```python
from build123d import *

# Parameters (mm, degrees)
F3_DEPTH  = 18.75
F4_W      = 19.4052183703
F4_H      = 18.75
F4_W_2    = 8
F5_DEPTH  = 3
F6_R      = 2.25
F7_DEPTH  = 12
F9_DEPTH  = 3.3
F11_DEPTH = 35


with BuildPart() as f3:
    # F2 (on Top) → F3 (new body)
    with BuildSketch(Plane.XY):
        Polygon((-6.6899931507, 11.2585633857), (-6.6899931507, 24.0085633857), (-5.1899931507, 24.0085633857), (-6.6899931507, 25.5085633857), (-9.6899931507, 25.5085633857), (-9.6899931507, 24.0085633857), (-9.6899931507, 11.2585633857), (-9.6899931507, -18.7414366143), (9.0600068493, -13.7414366143), (9.0600068493, 11.2585633857), (9.0600068493, 24.0085633857), (9.0600068493, 25.5085633857), (6.0600068493, 25.5085633857), (4.5600068493, 24.0085633857), (6.0600068493, 24.0085633857), (6.0600068493, 11.2585633857), align=None)
    extrude(amount=F3_DEPTH)

    # F4 (on face) → F5 (join)
    with BuildSketch(Plane(origin=(4.0225987819, -15.0847454323, 0), x_dir=(0.9662349396, 0.2576626506, 0), z_dir=(0.2576626506, -0.9662349396, 0))):
        with Locations((-4.4891689949, 9.375)):
            Rectangle(F4_W, F4_H)
        with Locations((-18.1917781801, 9.375)):
            Rectangle(F4_W_2, F4_H)
        with Locations((9.2134401902, 9.375)):
            Rectangle(F4_W_2, F4_H)
    extrude(amount=F5_DEPTH)

    # F6 (on face) → F7 (cut)
    with BuildSketch(Plane(origin=(4.7955867336, -17.9834502511, 0), x_dir=(0.9662349396, 0.2576626506, 0), z_dir=(0.2576626506, -0.9662349396, 0))):
        with Locations((7.2134401902, 9.375)):
            Circle(F6_R)
        with Locations((-16.1917781801, 9.375)):
            Circle(F6_R)
    extrude(amount=-F7_DEPTH, mode=Mode.SUBTRACT)

    # F8 (on face) → F9 (cut)
    with BuildSketch(Plane(origin=(4.0225987819, -15.0847454323, 0), x_dir=(0.9662349396, 0.2576626506, 0), z_dir=(0.2576626506, -0.9662349396, 0))):
        Polygon((5.2134401902, 5.775), (9.2919011593, 5.775), (11.3703621284, 9.375), (9.2919011593, 12.975), (5.2134401902, 12.975), align=None)
        Polygon((5.1349792211, 5.775), (5.2134401902, 5.775), (5.2134401902, 12.975), (5.1349792211, 12.975), (3.0565182521, 9.375), align=None)
        Polygon((-18.2702391492, 5.775), (-14.1917781801, 5.775), (-14.1917781801, 12.975), (-18.2702391492, 12.975), (-20.3487001183, 9.375), align=None)
        Polygon((-14.1917781801, 12.975), (-14.1917781801, 5.775), (-14.113317211, 5.775), (-12.0348562419, 9.375), (-14.113317211, 12.975), align=None)
    extrude(amount=-F9_DEPTH, mode=Mode.SUBTRACT)

    # F10 (on face) → F11 (join)
    with BuildSketch(Plane(origin=(0, 0, 0), x_dir=(1, 0, 0), z_dir=(0, 0, -1))):
        Polygon((9.0600068493, -8.2585633857), (-9.6899931507, -8.2585633857), (-9.6899931507, -25.5085633857), (-6.6899931507, -25.5085633857), (-5.1899931507, -24.0085633857), (-6.6899931507, -24.0085633857), (-6.6899931507, -11.2585633857), (6.0600068493, -11.2585633857), (6.0600068493, -24.0085633857), (4.5600068493, -24.0085633857), (6.0600068493, -25.5085633857), (9.0600068493, -25.5085633857), align=None)
    extrude(amount=F11_DEPTH)


solid = f3.part
```
Part model, mm, in its own coordinate system. A direction names the side the tool comes from. Round coordinates to 2 decimals unless told otherwise and drop trailing zeros. Loops run counter-clockwise (first coordinate to the right, second up) from the corner with the lowest first, then second, coordinate; pieces in that order, holes last.
Item 1: Mould opens along Y. For faces 1 (the face through (8.046, -4.697, 9.406)), 2 (the face through (0, 11, -35)), 3 (the face through (-5.95, 24.77, -7.75)), 4 (the face through (7.547, -12.461, 7.6)) say: +Y half, -Y half, draft (parallel to the pull), parting line (faces both ways), or undercut.
Item 2: Cut at A-A, the plane z = 15. Give the cut face in (x, y), then the cut area to 3 significant figures.
Item 3: Drop flat-ended pins along their axis: P1, Ø12, axis at y = -12, z = -9, coming from the -X side; P2, Ø1.6, axis at x = -6.5, z = -6.5, coming from the -Y side; P3, Ø0.7, axis at x = 8.5, y = -12.5, coming from the -Z side; P4, Ø4, axis at y = 15, z = -13.5, coming from the -X side. Give the stop position or say it passes through.
Item 4: Drill centre lines: line 1 (X direction, y = 14, z = 15.5); line 2 (Y direction, x = -7, z = -10); line 3 (Z direction, x = -1, y = -12). Where is each one in solid material? Low to high.
Item 5: 3-axis set-ups, long thin cutter, end or side, ignore diameter. For faces 5 (the face through (0, 11.259, -8)), 6 (the face through (17.17, -13.11, 9.24)), 7 (the face through (-8, 25.509, -8)), 8 (the face through (7.575, -12.454, 11.2)), 9 (the face through (0, 8.259, -17)): which of +Z, -Z, +X, -X, +Y, -Y reach the whole face in a straight line?
Item 6: Cut at B-B, the plane x = 3.5. Give the cut face in (y, z).
Item 7: Cut at C-C, the plane y = 5.5. Give the cut face in (x, z).
Item 8: Cut at D-D, the plane z = -14. Give the cut face in (x, y).
A:
1. face 1: undercut
1. face 2: draft
1. face 3: +Y half
1. face 4: undercut
2. outline: (-17.42, -20.8) - (-16.65, -23.7) - (17.56, -14.58) - (16.79, -11.68) - (9.06, -13.74) - (9.06, 25.51) - (6.06, 25.51) - (4.56, 24.01) - (6.06, 24.01) - (6.06, 11.26) - (-6.69, 11.26) - (-6.69, 24.01) - (-5.19, 24.01) - (-6.69, 25.51) - (-9.69, 25.51) - (-9.69, -18.74) - close
2. area: 710 mm2
3. P1: passes through
3. P2: stops at y = 8.26
3. P3: stops at z = 0
3. P4: stops at x = -9.69
4. line 1: x = -9.69 to -6.69, 6.06 to 9.06
4. line 2: y = 8.26 to 25.51
4. line 3: z = 0 to 18.75
5. face 5: +Z, -Z
5. face 6: +Z, -Z, +X, +Y
5. face 7: +Z, -Z, +X, -X, +Y
5. face 8: none
5. face 9: -Z, +X, -X, -Y
6. outline: (-18.33, 0) - (8.26, 0) - (8.26, -35) - (11.26, -35) - (11.26, 18.75) - (-18.33, 18.75) - close
7. outline: (-9.69, 0) - (9.06, 0) - (9.06, 18.75) - (-9.69, 18.75) - close
8. outline: (-9.69, 8.26) - (9.06, 8.26) - (9.06, 25.51) - (6.06, 25.51) - (4.56, 24.01) - (6.06, 24.01) - (6.06, 11.26) - (-6.69, 11.26) - (-6.69, 24.01) - (-5.19, 24.01) - (-6.69, 25.51) - (-9.69, 25.51) - close
